The drawing under review shows one solid part. Ordinate dimensions are in mm from its lowest x, y, z. Coordinates: 2 decimals unless noted, no trailing zeros. Loops run counter-clockwise (first coordinate to the right, second up) from the corner with the lowest first, then second, coordinate; pieces in that order, holes last. Notation, with made-up numbers: M 37,-26 L 53,-26 A9 cw 53,-22 Z; hole C 10,-7.75 d7. An arc over 180 degrees is marked long. Use one line per item in the form item = value.
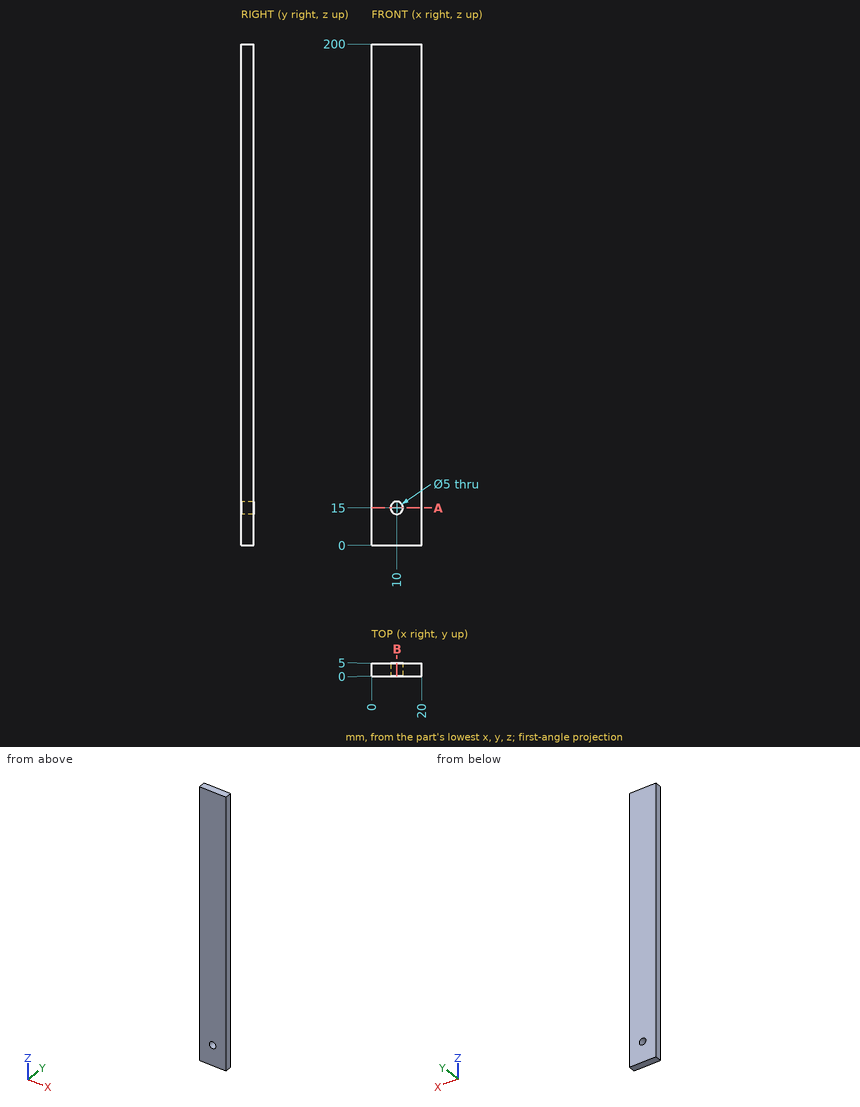
1. Consider section B-B on x = 10. Write out the cut boundary in (y, z).
Computed values:
outline = M 0,0 L 5,0 L 5,12.5 L 0,12.5 Z; M 0,17.5 L 5,17.5 L 5,200 L 0,200 Z
2. For pin 1 Ø6.5 at (x, z) = (10, 15) entering from -Y, flat-tipped, find the tip position at first contact; note if it passes through.
Computed values:
pin_1 = 0
3. Wall thickness on line 1 along Z through (x, y) = (10, 1.3); line 2 along Z through (x, y) = (9.5, 3.45): over which ranges is each line inside the solid? List them lowest first. Write a range as from..to.
Computed values:
line_1 = 0..12.5, 17.5..200
line_2 = 0..12.55, 17.45..200
4. Consider section A-A on z = 15. Write out the cut boundary in (x, y), plus the area to 3 significant figures.
Computed values:
outline = M 0,0 L 7.5,0 L 7.5,5 L 0,5 Z; M 12.5,0 L 20,0 L 20,5 L 12.5,5 Z
area = 75.0 mm2
